Could you check a few things on this model? Use its own coordinates, in mm. A direction names the side the tool comes from. Coordinates: 2 decimals unless noted, no trailing zeros. Order: outer loops, then holes, each group sorted by start corner. A loop starts at its lowest first (then second) coordinate and runs counter-clockwise, first axis right, second up. Notation, with made-up numbers: (81.25, 42.5) - (89.25, 42.5) arc R28 cw to (89.25, 63.5) - close; hole circle Ø8 at (-8, 44.25). An arc over 180 degrees is marked (long way). Answer as CSV lines item,"result". Start each with the question number.
1. I want a section at B-B, the plane y = 152.5. List the corners of the cut face in (x, z) for me, and give its area (3 significant figures).
2. I want a section at C-C, the plane z = 2.15. Count the separate pieces of the cut face and the enclosed holes in it, and give its area (3 significant figures).
3. I want a section at A-A, the plane x = 155.5. List the corners of the cut face in (y, z) for me.
4. I need wall thicknesses on probe 1 along Y at (x, z) = (104, 2); probe 2 along Y at (x, z) = (131.5, 0.2); probe 3 along X at (y, z) = (120, 0.8). Which ranges of each line are inside material? Lowest first, please.
5. For faces 4 (the face through (170, 156.112, 2)), 5 (the face through (135.671, 204, 2)), 6 (the face through (127.345, 104, 2)), 7 (the face through (165, 202.396, 2)), which set-ups out of +Z, -Z, +X, -X, +Y, -Y let a thin tool reach every point of the face, with its end or its side?
6. Thinking about a two-plate mould opening in X: for faces 1 (the face through (167.668, 136, 2)), 2 (the face through (170, 140.096, 2)), 3 (the face through (161.212, 113, 2)), which applies, released by +X, released by -X, zero draft, split by the parting line, or undercut?
7. For pin 1 (1.8 mm diameter, centred on y = 182.5, z = 2.5, fed in from -X); pin 2 (1.8 mm diameter, centred on x = 93.5, z = 2, fed in from -Y); pin 3 (2 mm diameter, centred on y = 155, z = 1, fed in from +X), each with a flat end and sliding along its axis, tell me the tip position at first contact or that it passes through.
from build123d import *

# Parameters (mm, degrees)
MODEL_W             = 59.689998908
MODEL_H             = 3.386668819
MODEL_H_2           = 3.386666801
BOSS_EXTRUDE1_DEPTH = 3.7


with BuildPart() as part:
    # Model → Boss-Extrude1 (new body)
    with BuildSketch(Plane.XY):
        Polygon((171.653953395, 180.763341901), (167.667564776, 180.763341901), (167.667564776, 188.523500843), (171.653953393, 188.523500843), (171.653953393, 196.849055858), (167.667564774, 196.849055858), (167.667564774, 202.396336528), (161.352865562, 202.396336528), (161.352865562, 206.382725147), (151.651476676, 206.382725147), (151.651476676, 202.396336528), (143.3611989, 202.396336528), (143.3611989, 206.382725147), (135.670644961, 206.382725147), (135.670644961, 202.396336528), (127.3450886, 202.396336528), (127.3450886, 206.382725147), (119.654533316, 206.382725147), (119.654533316, 202.396336528), (111.36425554, 202.396336528), (111.36425554, 206.382725147), (101.662866654, 206.382725147), (101.662866654, 202.396336528), (95.348117657, 202.396336528), (95.348117657, 196.809013257), (91.361729039, 196.809013257), (91.361729039, 188.483458242), (95.348117657, 188.483458848), (95.348117657, 180.418280574), (91.361733076, 180.418280574), (91.361733076, 172.092725559), (95.348117657, 172.092725559), (95.348117657, 164.402168929), (91.361733076, 164.402168929), (91.361733076, 156.111891153), (95.348117657, 156.111891153), (95.348117657, 148.421337214), (91.361733076, 148.421337214), (91.361733076, 140.095782199), (95.348117657, 140.095782199), (95.348117657, 132.405225569), (91.361733076, 132.405225569), (91.361733076, 124.114947793), (95.348117574, 124.114947793), (95.348117574, 116.440193769), (91.361728955, 116.440193769), (91.361728955, 107.667091645), (95.348117574, 107.667091645), (95.348117658, 102.101616643), (101.662843109, 102.101616643), (101.662843109, 106.123281156), (111.364231995, 106.123281156), (111.364231995, 102.101616643), (119.654509771, 102.101616643), (119.654509771, 106.123281156), (127.34506371, 106.123281156), (127.34506371, 102.101616643), (135.67062007, 102.101616643), (135.67062007, 106.123281156), (143.361175355, 106.123281156), (143.361175355, 102.101616643), (151.651453131, 102.101616643), (151.651453131, 106.123281156), (161.352842017, 106.123281156), (161.352842017, 102.101616643), (167.820439872, 102.103733493), (167.820439872, 107.429661364), (171.653953395, 107.429661364), (171.653953395, 116.049769541), (167.667564776, 116.049769541), (167.667564776, 123.789730804), (171.653953395, 123.789730804), (171.653953395, 132.405225594), (167.667564776, 132.405225594), (167.667564776, 136.4004416), (167.667564776, 140.095782224), (171.653953395, 140.095782224), (171.653953395, 148.421337239), (167.667564776, 148.421337239), (167.667564776, 153.3044818), (167.667564776, 156.111891178), (171.653953395, 156.111891178), (171.653953395, 164.402168953), (167.667564776, 164.402168953), (167.667564776, 172.092725584), (171.653953395, 172.092725584), align=None)
        with Locations((131.366728222, 112.565500146)):
            Rectangle(MODEL_W, MODEL_H, mode=Mode.SUBTRACT)
        with Locations((131.366728222, 192.567447735)):
            Rectangle(MODEL_W, MODEL_H_2, mode=Mode.SUBTRACT)
    extrude(amount=BOSS_EXTRUDE1_DEPTH)


solid = part.part
Solved:
1,outline,"(95.35, 0) - (167.67, 0) - (167.67, 3.7) - (95.35, 3.7) - close"
1,area,"268 mm2"
2,separate pieces,"1"
2,enclosed holes,"2"
2,area,"7,250 mm2"
3,outline,"(106.12, 0) - (110.87, 0) - (110.87, 3.7) - (106.12, 3.7) - close; (114.26, 0) - (190.87, 0) - (190.87, 3.7) - (114.26, 3.7) - close; (194.26, 0) - (206.38, 0) - (206.38, 3.7) - (194.26, 3.7) - close"
4,probe 1,"y = 106.12 to 110.87, 114.26 to 190.87, 194.26 to 206.38"
4,probe 2,"y = 102.1 to 110.87, 114.26 to 190.87, 194.26 to 202.4"
4,probe 3,"x = 95.35 to 167.67"
5,face 4,"+Z, -Z, +X"
5,face 5,"+Z, -Z, +Y"
5,face 6,"+Z, -Z, -Y"
5,face 7,"+Z, -Z, +X, +Y"
6,face 1,"released by +X"
6,face 2,"zero draft"
6,face 3,"undercut"
7,pin 1,"stops at x = 95.35"
7,pin 2,"stops at y = 107.67"
7,pin 3,"stops at x = 167.67"
